from build123d import *

# Parameters (mm, degrees)
SKETCH1_R           = 19.05
BOSS_EXTRUDE1_DEPTH = 12.7
SKETCH2_R           = 3.175
CUT_EXTRUDE1_DEPTH  = 17.78
SKETCH3_R           = 6.35
CUT_EXTRUDE2_DEPTH  = 3.175
SKETCH4_R           = 4.445
CUT_EXTRUDE3_DEPTH  = 38.1
SKETCH5_R           = 6.604
CUT_EXTRUDE4_DEPTH  = 6.35


with BuildPart() as part:
    # Sketch1 → Boss-Extrude1 (new body)
    with BuildSketch(Plane(origin=(0, 0, 0), x_dir=(1, 0, 0), z_dir=(0, 1, 0))):
        with Locations(Location((0, 0, 0), (0, 0, 270))):
            Circle(SKETCH1_R)
    extrude(amount=-BOSS_EXTRUDE1_DEPTH)

    # Sketch2 → Cut-Extrude1 (cut)
    with BuildSketch(Plane(origin=(0, 0, 0), x_dir=(1, 0, 0), z_dir=(0, 1, 0))):
        with Locations(Location((0, 0, 0), (0, 0, 270))):
            Circle(SKETCH2_R)
    extrude(amount=-CUT_EXTRUDE1_DEPTH, mode=Mode.SUBTRACT)

    # Sketch3 → Cut-Extrude2 (cut)
    with BuildSketch(Plane(origin=(0, 0, 0), x_dir=(1, 0, 0), z_dir=(0, 1, 0))):
        with Locations(Location((0, 0, 0), (0, 0, 270))):
            Circle(SKETCH3_R)
    extrude(amount=-CUT_EXTRUDE2_DEPTH, mode=Mode.SUBTRACT)

    # Sketch4 → Cut-Extrude3 (cut)
    with BuildSketch(Plane(origin=(0, 0, 0), x_dir=(1, 0, 0), z_dir=(0, 1, 0))):
        with Locations(Location((-2.346030642, 11.648567038, 0), (0, 0, 270))):
            Circle(SKETCH4_R)
    extrude(amount=-CUT_EXTRUDE3_DEPTH, mode=Mode.SUBTRACT)

    # Sketch5 → Cut-Extrude4 (cut)
    with BuildSketch(Plane(origin=(0, -12.7, 0), x_dir=(1, 0, 0), z_dir=(0, 1, 0))):
        with Locations((-13.400281264, 17.901049998)):
            Circle(SKETCH5_R)
    extrude(amount=CUT_EXTRUDE4_DEPTH, mode=Mode.SUBTRACT)


solid = part.part
Could you check a few things on this model? Use its own coordinates, in mm. A direction names the side the tool comes from. Round coordinates to 2 decimals unless told otherwise and drop trailing zeros. Order: outer loops, then holes, each group sorted by start corner. A loop starts at its lowest first (then second) coordinate and runs counter-clockwise, first axis right, second up.
Q1. Which directions (+Z, -Z, +X, -X, +Y, -Y) give clear straight access to the entire face, cutting with the end or side of a thin tool? Please do faces 1 (the face through (3, -3.175, -2)), 2 (the face through (5.72, -6.26, 18.17)).
Geometry says:
face 1: +Y
face 2: +Y, -Y
Q2. Imagine slicing it at D-D, the plane z = -13. List the corners of the cut face in (x, y) for me, then the cut area to 3 significant figures.
Geometry says:
outline: (-13.92, -6.35) - (-8.97, -6.35) - (-8.97, -12.7) - (-6.58, -12.7) - (-6.58, 0) - (-13.92, 0) - close; (1.89, -12.7) - (13.92, -12.7) - (13.92, 0) - (1.89, 0) - close
area: 215 mm2
Q3. Imagine slicing it at A-A, the plane z = 0. List the corners of the cut face in (x, y) for me (3 decimals), then the cut area to 3 significant figures.
Geometry says:
outline: (-19.05, -12.7) - (-3.175, -12.7) - (-3.175, -3.175) - (-6.35, -3.175) - (-6.35, 0) - (-19.05, 0) - close; (3.175, -12.7) - (19.05, -12.7) - (19.05, 0) - (6.35, 0) - (6.35, -3.175) - (3.175, -3.175) - close
area: 383 mm2
Q4. Imagine slicing it at B-B, the plane x = 0. List the corners of the cut face in (y, z) for me (3 decimals), then the cut area to 3 significant figures.
Geometry says:
outline: (-12.7, -19.05) - (0, -19.05) - (0, -15.424) - (-12.7, -15.424) - close; (-12.7, -7.873) - (0, -7.873) - (0, -6.35) - (-3.175, -6.35) - (-3.175, -3.175) - (-12.7, -3.175) - close; (-12.7, 3.175) - (-3.175, 3.175) - (-3.175, 6.35) - (0, 6.35) - (0, 19.05) - (-12.7, 19.05) - close
area: 287 mm2
Q5. Imagine slicing it at C-C, the plane y = -8. List the corners of the cut face in (x, z) for me (3 decimals), then the cut area to 3 significant figures.
Geometry says:
outline: (-15.16, -11.536) arc R6.604 cw to (-6.797, -17.796) arc R19.05 ccw (long way) to start; hole circle Ø8.89 at (-2.346, -11.649); hole circle Ø6.35 at (0, 0)
area: 1,020 mm2
Q6. I'm going to push flat-ended pins straight in: P1, Ø10, axis at x = 0, z = 0, coming from the -Y side; P2, Ø4, axis at x = 15, y = -5.5, coming from the -Z side; P3, Ø2, axis at y = -8.5, z = 6.5, coming from the -X side; P4, Ø6, axis at x = 6.5, y = -4.5, coming from the +Z side. Where does each tip first touch, or does it pass through?
Geometry says:
P1: stops at y = -12.7
P2: stops at z = -13.92
P3: stops at x = -18.24
P4: stops at z = 18.73
Q7. Please list where these lines run through material, in increasing order: probe 1 along X at (y, z) = (-3.75, -14.5); probe 2 along X at (y, z) = (-11.25, -1); probe 3 along Y at (x, z) = (0.5, 4) (3 decimals).
Geometry says:
probe 1: x = -12.36 to -5.76, 1.06 to 12.36
probe 2: x = -19.02 to -3.01, 3.01 to 19.02
probe 3: y = -12.7 to -3.175
Q8. Thinking about a two-plate mould opening in Z: for faces 3 (the face through (-10, -6.35, -14)), 4 (the face through (-1.93, -7.87, -2.52)), 5 (the face through (-3.86, -1.57, -5.04)), 6 (the face through (-9.511, -9.569, -12.564)), which applies, released by +Z, released by -Z, zero draft, split by the parting line, or undercut?
Geometry says:
face 3: zero draft
face 4: undercut
face 5: undercut
face 6: released by -Z
